from build123d import *

# Parameters (mm, degrees)
F1_DEPTH = 25.4
F3_DEPTH = 25.4


with BuildPart() as f1:
    # F0 (on Front) → F1 (new body)
    with BuildSketch(Plane.XZ):
        Polygon((38.1, 56.983866), (0, 0), (76.2, 0), align=None)
    extrude(amount=F1_DEPTH)

    # F2 (on face) → F3 (cut)
    with BuildSketch(Plane.XZ.offset(25.4)):
        with BuildLine():
            ThreePointArc((50.127231, 23.25872), (29.595463, 31.763256), (38.1, 11.231488))
            ThreePointArc((38.1, 11.231488), (46.604537, 14.754183), (50.127231, 23.25872))
        make_face()
    extrude(amount=-F3_DEPTH, mode=Mode.SUBTRACT)


solid = f1.part
Work out the finished part from the listing and answer in its coordinate system (mm). Give positions to 0.01 mm unless a question says otherwise; leave off trailing zeros. Order: outer loops, then holes, each group sorted by start corner. A loop starts at its lowest first (then second) coordinate and runs counter-clockwise, first axis right, second up. Notation, with made-up numbers: (77.5, 81) -> (121.5, 81) arc R28 cw to (121.5, 110) -> close; hole circle Ø3 at (65, 50). An arc over 180 degrees is marked (long way). Answer as a JSON object with one key per item and string values. Group by question number.
1. Section B-B on y = -3 is taken. Determine the outline of the cut face in (x, z), plus the area to 3 significant figures.
2. Section D-D on z = 45.5 is taken. Determine the outline of the cut face in (x, y), plus the area to 3 significant figures.
3. The mould has two halves that part along X. Classify faces 1 (the flat face through (19.317, -12.522, 28.891)), 2 (the flat face through (38, -25.4, 10)), 3 (the flat face through (57.42, -12.52, 28.09)): released by +X, released by -X, zero draft, split by the parting line, or undercut.
4. Section C-C on z = 18 is taken. Determine the outline of the cut face in (x, y).
5. Consider line 1 along X through (y, z) = (-5.5, 28.5); line 2 along Z through (x, y) = (41.5, -10.5); line 3 along X through (y, z) = (-14.5, 14.5). Determine where each line is inside the solid, lowest interval first. Write a range as [from, to].
6. Flat-ended cylindrical pins translate along their axes: pin 1 Ø6 at (y, z) = (-19.5, 39) entering from +X; pin 2 Ø2 at (y, z) = (-3, 22) entering from +X; pin 3 Ø1.5 at (y, z) = (-9, 43.5) entering from +X. Find the tip coordinate at first contact, or state that the pin passes through.
7. Section A-A on x = 35 is taken. Determine the outline of the cut face in (y, z), plus the area to 3 significant figures.
Result sheet:
{
 "1": {"outline": "(0, 0) -> (76.2, 0) -> (38.1, 56.98) -> close; hole circle Ø24.05 at (38.1, 23.26)", "area": "1,720 mm^2"},
 "2": {"outline": "(30.42, -25.4) -> (45.78, -25.4) -> (45.78, 0) -> (30.42, 0) -> close", "area": "390 mm^2"},
 "3": {"face 1": "released by -X", "face 2": "zero draft", "face 3": "released by +X"},
 "4": {"outline": "(12.03, -25.4) -> (27.28, -25.4) -> (27.28, 0) -> (12.03, 0) -> close; (48.92, -25.4) -> (64.17, -25.4) -> (64.17, 0) -> (48.92, 0) -> close"},
 "5": {"line 1": "x = [19.06, 27.27], [48.93, 57.14]", "line 2": "z = [0, 11.72], [34.8, 51.9]", "line 3": "x = [9.69, 29.86], [46.34, 66.51]"},
 "6": {"pin 1": "stops at x = 52.13", "pin 2": "stops at x = 62.16", "pin 3": "stops at x = 47.62"},
 "7": {"outline": "(-25.4, 0) -> (0, 0) -> (0, 11.64) -> (-25.4, 11.64) -> close; (-25.4, 34.88) -> (0, 34.88) -> (0, 52.35) -> (-25.4, 52.35) -> close", "area": "739 mm^2"}
}
